Build history of the part. All positions in model axes, mm. Round coordinates to 2 decimals unless told otherwise and drop trailing zeros. Order: outer loops, then holes, each group sorted by start corner. A loop starts at its lowest first (then second) coordinate and runs counter-clockwise, first axis right, second up. Notation, with made-up numbers: (49.25, 55) -> (62.25, 55) arc R21 ccw to (62.25, 77) -> close; hole circle Ø7 at (48, -7). An arc over 180 degrees is marked (long way). Answer as CSV lines item,"result". Start each with the question number.
```python
from build123d import *

# Parameters (mm, degrees)
TOOTH_DEPTH         = 6.35
CIRPATTERN2_COUNT   = 14
FILLET2_R           = 1.27
CIRPATTERN10_DEPTH  = 6.35
SKETCH2_R           = 44.45
SKETCH2_R_2         = 3.175
SKETCH2_R_3         = 33.655
BOSS_EXTRUDE2_DEPTH = 6.35


# Read off the part's stored shape, not the designer's step: CirPattern10
with BuildPart() as part:
    # Sketch1 → tooth (new body)
    with BuildSketch(Plane(origin=(0, 0, 0), x_dir=(1, 0, 0), z_dir=(0, 1, 0))):
        with BuildLine():
            Line((23.495, 1.905), (27.019279154, 3.939743518))
            ThreePointArc((27.019279154, 3.939743518), (26.594581963, 6.18799121), (25.983150393, 8.392789801))
            Line((25.983150393, 8.392789801), (32.025743508, 10.344601382))
            ThreePointArc((32.025743508, 10.344601382), (33.536845379, 2.817627907), (33.302832446, -4.855962941))
            Line((33.302832446, -4.855962941), (27.019279154, -3.939743518))
            Line((27.019279154, -3.939743518), (23.495, -1.905))
            ThreePointArc((23.495, -1.905), (23.572103215, 0), (23.495, 1.905))
        make_face()
    tooth = extrude(amount=TOOTH_DEPTH)

    # CirPattern2: tooth ×14 about axis
    cirpattern2_axis = Axis((0, 0, 0), (0, 1, 0))
    for i in range(1, CIRPATTERN2_COUNT):
        add(tooth.rotate(cirpattern2_axis, i * 360 / CIRPATTERN2_COUNT))

    # Fillet2
    fillet2_edges = [part.edges().sort_by_distance(p)[0] for p in [
        (20.341715028, 3.175, -11.910444144),
        (21.994812074, 3.175, -8.477752757),
    ]]
    fillet(fillet2_edges, radius=FILLET2_R)

    # CirPattern10 outline → CirPattern10 (cut)
    with BuildSketch(Plane(origin=(0, 0, 0), x_dir=(1, 0, 0), z_dir=(0, 1, 0))):
        with BuildLine():
            ThreePointArc((21.994812074, -8.477752757), (21.853716341, -8.835107925), (21.706815016, -9.190115986))
            ThreePointArc((21.706815016, -9.190115986), (22.135768899, -8.653514623), (22.781411207, -8.418805301))
            Line((22.781411207, -8.418805301), (21.994812074, -8.477752757))
        make_face()
        with BuildLine():
            ThreePointArc((20.786064589, -12.562185248), (20.567016331, -11.911062896), (20.719099799, -11.241127769))
            ThreePointArc((20.719099799, -11.241127769), (20.533134799, -11.577323755), (20.341715028, -11.910444144))
            Line((20.341715028, -11.910444144), (20.786064589, -12.562185248))
        make_face()
        with BuildLine():
            ThreePointArc((16.138281869, -17.181382608), (15.85610841, -17.442129345), (15.569722665, -17.698242459))
            ThreePointArc((15.569722665, -17.698242459), (16.189019364, -17.400897451), (16.872559541, -17.469565358))
            Line((16.872559541, -17.469565358), (16.138281869, -17.181382608))
        make_face()
        with BuildLine():
            ThreePointArc((13.277069174, -20.336873246), (13.362224913, -19.655190801), (13.789921341, -19.117586652))
            ThreePointArc((13.789921341, -19.117586652), (13.476502695, -19.339801579), (13.159503921, -19.556878753))
            Line((13.159503921, -19.556878753), (13.277069174, -20.336873246))
        make_face()
        with BuildLine():
            ThreePointArc((7.085367016, -22.482028918), (6.718003745, -22.594523135), (6.348855789, -22.70101496))
            ThreePointArc((6.348855789, -22.70101496), (7.035835999, -22.701819131), (7.62189053, -23.060263746))
            Line((7.62189053, -23.060263746), (7.085367016, -22.482028918))
        make_face()
        with BuildLine():
            ThreePointArc((3.138387377, -24.083594083), (3.510880975, -23.506367113), (4.12947984, -23.207573037))
            ThreePointArc((4.12947984, -23.207573037), (3.750683953, -23.271794514), (3.370891671, -23.329833676))
            Line((3.370891671, -23.329833676), (3.138387377, -24.083594083))
        make_face()
        with BuildLine():
            ThreePointArc((-3.370891671, -23.329833676), (-3.750683953, -23.271794514), (-4.12947984, -23.207573037))
            ThreePointArc((-4.12947984, -23.207573037), (-3.510880975, -23.506367113), (-3.138387377, -24.083594083))
            Line((-3.138387377, -24.083594083), (-3.370891671, -23.329833676))
        make_face()
        with BuildLine():
            ThreePointArc((-7.62189053, -23.060263746), (-7.035835999, -22.701819131), (-6.348855789, -22.701014959))
            ThreePointArc((-6.348855789, -22.701014959), (-6.718003745, -22.594523135), (-7.085367016, -22.482028918))
            Line((-7.085367016, -22.482028918), (-7.62189053, -23.060263746))
        make_face()
        with BuildLine():
            ThreePointArc((-13.159503921, -19.556878753), (-13.476502695, -19.339801579), (-13.789921341, -19.117586652))
            ThreePointArc((-13.789921341, -19.117586652), (-13.362224913, -19.655190801), (-13.277069174, -20.336873246))
            Line((-13.277069174, -20.336873246), (-13.159503921, -19.556878753))
        make_face()
        with BuildLine():
            ThreePointArc((-16.872559541, -17.469565358), (-16.189019364, -17.400897451), (-15.569722665, -17.698242459))
            ThreePointArc((-15.569722665, -17.698242459), (-15.85610841, -17.442129345), (-16.138281869, -17.181382608))
            Line((-16.138281869, -17.181382608), (-16.872559541, -17.469565358))
        make_face()
        with BuildLine():
            ThreePointArc((-20.341715028, -11.910444144), (-20.533134799, -11.577323755), (-20.719099799, -11.241127769))
            ThreePointArc((-20.719099799, -11.241127769), (-20.567016331, -11.911062896), (-20.786064589, -12.562185248))
            Line((-20.786064589, -12.562185248), (-20.341715028, -11.910444144))
        make_face()
        with BuildLine():
            ThreePointArc((-22.781411207, -8.418805301), (-22.135768899, -8.653514623), (-21.706815017, -9.190115986))
            ThreePointArc((-21.706815017, -9.190115986), (-21.853716341, -8.835107925), (-21.994812074, -8.477752757))
            Line((-21.994812074, -8.477752757), (-22.781411207, -8.418805301))
        make_face()
        with BuildLine():
            ThreePointArc((-23.495, -1.905), (-23.522927734, -1.521814974), (-23.544606438, -1.138225668))
            ThreePointArc((-23.544606438, -1.138225668), (-23.698257926, -1.807802905), (-24.178124988, -2.299402395))
            Line((-24.178124988, -2.299402395), (-23.495, -1.905))
        make_face()
        with BuildLine():
            ThreePointArc((-24.178124988, 2.299402395), (-23.698257926, 1.807802905), (-23.544606438, 1.138225668))
            ThreePointArc((-23.544606438, 1.138225668), (-23.522927734, 1.521814974), (-23.495, 1.905))
            Line((-23.495, 1.905), (-24.178124988, 2.299402395))
        make_face()
        with BuildLine():
            ThreePointArc((-21.994812074, 8.477752757), (-21.853716341, 8.835107925), (-21.706815016, 9.190115986))
            ThreePointArc((-21.706815016, 9.190115986), (-22.135768899, 8.653514623), (-22.781411207, 8.418805301))
            Line((-22.781411207, 8.418805301), (-21.994812074, 8.477752757))
        make_face()
        with BuildLine():
            ThreePointArc((-20.786064589, 12.562185248), (-20.567016331, 11.911062896), (-20.719099799, 11.241127769))
            ThreePointArc((-20.719099799, 11.241127769), (-20.533134799, 11.577323755), (-20.341715028, 11.910444144))
            Line((-20.341715028, 11.910444144), (-20.786064589, 12.562185248))
        make_face()
        with BuildLine():
            ThreePointArc((-16.138281869, 17.181382608), (-15.85610841, 17.442129345), (-15.569722665, 17.698242459))
            ThreePointArc((-15.569722665, 17.698242459), (-16.189019364, 17.400897451), (-16.872559541, 17.469565358))
            Line((-16.872559541, 17.469565358), (-16.138281869, 17.181382608))
        make_face()
        with BuildLine():
            ThreePointArc((-13.277069174, 20.336873246), (-13.362224913, 19.655190801), (-13.789921341, 19.117586652))
            ThreePointArc((-13.789921341, 19.117586652), (-13.476502695, 19.339801579), (-13.159503921, 19.556878753))
            Line((-13.159503921, 19.556878753), (-13.277069174, 20.336873246))
        make_face()
        with BuildLine():
            ThreePointArc((-7.085367016, 22.482028918), (-6.718003745, 22.594523135), (-6.348855789, 22.70101496))
            ThreePointArc((-6.348855789, 22.70101496), (-7.035835999, 22.701819131), (-7.62189053, 23.060263746))
            Line((-7.62189053, 23.060263746), (-7.085367016, 22.482028918))
        make_face()
        with BuildLine():
            ThreePointArc((-3.138387377, 24.083594083), (-3.510880975, 23.506367113), (-4.12947984, 23.207573037))
            ThreePointArc((-4.12947984, 23.207573037), (-3.750683953, 23.271794514), (-3.370891671, 23.329833676))
            Line((-3.370891671, 23.329833676), (-3.138387377, 24.083594083))
        make_face()
        with BuildLine():
            ThreePointArc((3.370891671, 23.329833676), (3.750683953, 23.271794514), (4.12947984, 23.207573037))
            ThreePointArc((4.12947984, 23.207573037), (3.510880975, 23.506367113), (3.138387377, 24.083594083))
            Line((3.138387377, 24.083594083), (3.370891671, 23.329833676))
        make_face()
        with BuildLine():
            ThreePointArc((7.62189053, 23.060263746), (7.035835999, 22.701819131), (6.348855789, 22.701014959))
            ThreePointArc((6.348855789, 22.701014959), (6.718003745, 22.594523135), (7.085367016, 22.482028918))
            Line((7.085367016, 22.482028918), (7.62189053, 23.060263746))
        make_face()
        with BuildLine():
            ThreePointArc((13.159503921, 19.556878753), (13.476502695, 19.339801579), (13.789921341, 19.117586652))
            ThreePointArc((13.789921341, 19.117586652), (13.362224913, 19.655190801), (13.277069174, 20.336873246))
            Line((13.277069174, 20.336873246), (13.159503921, 19.556878753))
        make_face()
        with BuildLine():
            ThreePointArc((16.872559541, 17.469565358), (16.189019364, 17.400897451), (15.569722665, 17.698242459))
            ThreePointArc((15.569722665, 17.698242459), (15.85610841, 17.442129345), (16.138281869, 17.181382608))
            Line((16.138281869, 17.181382608), (16.872559541, 17.469565358))
        make_face()
        with BuildLine():
            ThreePointArc((23.495, 1.905), (23.522927734, 1.521814974), (23.544606438, 1.138225668))
            ThreePointArc((23.544606438, 1.138225668), (23.698257926, 1.807802905), (24.178124988, 2.299402395))
            Line((24.178124988, 2.299402395), (23.495, 1.905))
        make_face()
        with BuildLine():
            ThreePointArc((24.178124988, -2.299402395), (23.698257926, -1.807802905), (23.544606438, -1.138225668))
            ThreePointArc((23.544606438, -1.138225668), (23.522927734, -1.521814974), (23.495, -1.905))
            Line((23.495, -1.905), (24.178124988, -2.299402395))
        make_face()
    extrude(amount=CIRPATTERN10_DEPTH, mode=Mode.SUBTRACT)

    # Sketch2 → Boss-Extrude2 (add)
    with BuildSketch(Plane.XZ):
        with Locations(Location((0, 0, 0), (0, 0, 270))):
            Circle(SKETCH2_R)
        with Locations(Location((38.1, 0, 0), (0, 0, 270))):
            Circle(SKETCH2_R_2, mode=Mode.SUBTRACT)
        Circle(SKETCH2_R_3, mode=Mode.SUBTRACT)
        with Locations(Location((19.05, -32.995567884, 0), (0, 0, 270))):
            Circle(SKETCH2_R_2, mode=Mode.SUBTRACT)
        with Locations(Location((-19.05, -32.995567884, 0), (0, 0, 270))):
            Circle(SKETCH2_R_2, mode=Mode.SUBTRACT)
        with Locations(Location((-38.1, 0, 0), (0, 0, 270))):
            Circle(SKETCH2_R_2, mode=Mode.SUBTRACT)
        with Locations(Location((-19.05, 32.995567884, 0), (0, 0, 270))):
            Circle(SKETCH2_R_2, mode=Mode.SUBTRACT)
        with Locations(Location((19.05, 32.995567884, 0), (0, 0, 270))):
            Circle(SKETCH2_R_2, mode=Mode.SUBTRACT)
    extrude(amount=-BOSS_EXTRUDE2_DEPTH)


solid = part.part
```
Q1. Two-plate mould, pull along X, no slides. Class faces 1 (the face through (37.48, 3.13, -23.9)), 2 (the face through (17.834, 3.131, -35.928)), 3 (the face through (-19, 6.35, -19)): +X half, -X half, draft (parallel to the pull), parting line (faces both ways), or undercut.
Q2. Slice it at A-A, the plane x = 0. Write the cut outline in (y, z) (3 decimals).
Q3. Probe L1, parallel to Z at x = -22.5, y = 1; L2, parallel to X at y = 2.5, z = 33.5; L3, parallel to X at y = 4.5, z = 2. List the from-to ranges inside material, lowest first.
Q4. Slice it at B-B, the plane z = 0. Write the cut outline in (x, y) (3 decimals), plus the area to 3 significant figures.
Q5. Slice it at C-C, the plane z = -33.5. Write the cut outline in (x, y), plus the area to 3 significant figures.
Q6. Flat gauge pins, fed straight in: pin 1 Ø2 at (y, z) = (3.5, -7.5) entering from +X; pin 2 Ø2 at (y, z) = (1.5, 21.5) entering from -X; pin 3 Ø4 at (x, z) = (19.05, 33) entering from -Y; pin 4 Ø3 at (y, z) = (3, 29) entering from -X. Where does each tip first touch, or does it go through?
Q7. Slice it at D-D, the plane y = 4.75. Count the separate pieces of the cut face and the enclosed holes in it, plus the area to 3 significant figures.
Solutions:
1,face 1,"parting line"
1,face 2,"undercut"
1,face 3,"draft"
2,outline,"(0, -44.45) -> (6.35, -44.45) -> (6.35, -27.305) -> (0, -27.305) -> close; (0, 27.305) -> (6.35, 27.305) -> (6.35, 44.45) -> (0, 44.45) -> close"
3,L1,"z = -38.33 to -15.47, -15.08 to -8.47, 8.47 to 15.08, 15.47 to 38.33"
3,L2,"x = -29.22 to -22.18, -15.92 to 15.92, 22.18 to 29.22"
3,L3,"x = -44.4 to -40.57, -35.63 to -23.83, 23.83 to 35.63, 40.57 to 44.4"
4,outline,"(-44.45, 0) -> (-41.275, 0) -> (-41.275, 6.35) -> (-44.45, 6.35) -> close; (-34.925, 0) -> (-23.572, 0) -> (-23.572, 6.35) -> (-34.925, 6.35) -> close; (23.572, 0) -> (34.925, 0) -> (34.925, 6.35) -> (23.572, 6.35) -> close; (41.275, 0) -> (44.45, 0) -> (44.45, 6.35) -> (41.275, 6.35) -> close"
4,area,"185 mm2"
5,outline,"(-29.22, 0) -> (-22.18, 0) -> (-22.18, 6.35) -> (-29.22, 6.35) -> close; (-15.92, 0) -> (15.92, 0) -> (15.92, 6.35) -> (-15.92, 6.35) -> close; (22.18, 0) -> (29.22, 0) -> (29.22, 6.35) -> (22.18, 6.35) -> close"
5,area,"291 mm2"
6,pin 1,"stops at x = 43.97"
6,pin 2,"stops at x = -39.44"
6,pin 3,"passes through"
6,pin 4,"stops at x = -34.92"
7,separate pieces,"1"
7,enclosed holes,"7"
7,area,"3,980 mm2"
